Could you check a few things on this model? Use its own coordinates, in mm. Face numbers are marked on the shaded views. Round coordinates to 2 decimals unless told otherwise and drop trailing zeros. Loops run counter-clockwise (first coordinate to the right, second up) from the corner with the lowest first, then second, coordinate; pieces in that order, holes last. Notation, with made-up numbers: (10, 26) -> (18, 26) arc R29 cw to (18, 57) -> close; hole circle Ø9 at (-13, -28.5). An arc over 180 degrees is marked (long way). Put each result on its own line as item: value. Start each with the question number.
1. Imagine slicing it at A-A, the plane x = 3. Please give me the cut outline in (y, z) (3 decimals).
2. If we mould it in two halves opening along Z, with no side actions, what happens to the marked faces 1, 2 and 3? For each: pulls with the +Z half, pulls with the -Z half, needs draft (parallel to the pull), parting line crosses it, or undercut.
3. I need wall thicknesses on line 1 (Y direction, x = 1.9, z = 0) (3 decimals); line 2 (Y direction, x = 1.65, z = 1); line 3 (Z direction, x = 4.15, y = 0.25). Which ranges of each line are inside material? Lowest first, please. Write a range as [from, to].
4. I'm going to push flat-ended pins straight in: P1, Ø1, axis at x = 3.5, z = 0.5, coming from the +Y side; P2, Ø2, axis at x = 3.5, y = 1, coming from the +Z side; P3, Ø2, axis at x = 3.5, z = 2.5, coming from the -Y side; P4, Ø5, axis at y = 0, z = 0, coming from the +X side. Where does each tip first touch, or does it pass through?
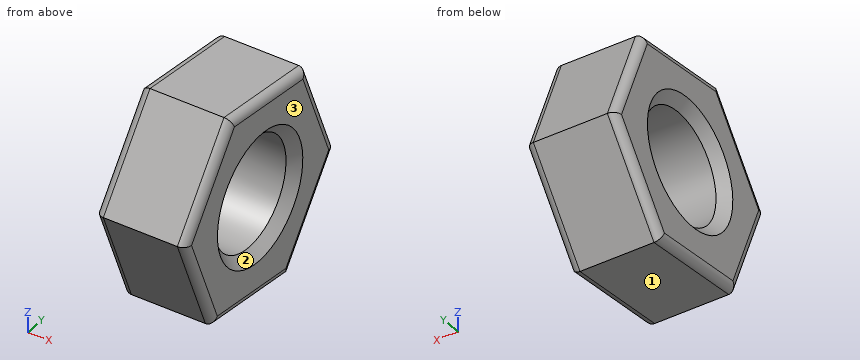
```python
from build123d import *

# Parameters (mm, degrees)
SKETCH1_R           = 2.705
BOSS_EXTRUDE1_DEPTH = 4.45
CHAMFER1_SIZE       = 0.5
FILLET1_R           = 0.4


with BuildPart() as part:
    # Sketch1 → Boss-Extrude1 (new body)
    with BuildSketch(Plane(origin=(0, 0, 0), x_dir=(0, 0, -1), z_dir=(1, 0, 0))):
        Polygon((0.806629144, 5.606072549), (-4.451686671, 3.501597604), (-5.258315815, -2.104474945), (-0.806629144, -5.606072549), (4.451686671, -3.501597604), (5.258315815, 2.104474945), align=None)
        Circle(SKETCH1_R, mode=Mode.SUBTRACT)
    extrude(amount=BOSS_EXTRUDE1_DEPTH)

    # Chamfer1
    chamfer1_edges = [part.edges().sort_by_distance(p)[0] for p in [
        (0, 0, 2.705),
        (4.45, 0, 2.705),
    ]]
    chamfer(chamfer1_edges, length=CHAMFER1_SIZE)

    # Fillet1
    fillet1_edges = [part.edges().sort_by_distance(p)[0] for p in [
        (4.45, 0.69856133, 4.855001243),
        (4.45, -3.855273747, 3.032472479),
        (4.45, -4.553835077, -1.822528764),
        (4.45, -0.69856133, -4.855001243),
        (4.45, 3.855273747, -3.032472479),
        (0, -0.69856133, -4.855001243),
        (0, -4.553835077, -1.822528764),
        (0, -3.855273747, 3.032472479),
        (0, 0.69856133, 4.855001243),
        (0, 4.553835077, 1.822528764),
        (0, 3.855273747, -3.032472479),
        (4.45, 4.553835077, 1.822528764),
    ]]
    fillet(fillet1_edges, radius=FILLET1_R)


solid = part.part
```
Entries:
1. outline: (-5.606, 0.807) -> (-3.502, -4.452) -> (2.104, -5.258) -> (5.606, -0.807) -> (3.502, 4.452) -> (-2.104, 5.258) -> close; hole circle Ø5.41 at (0, 0)
2. face 1: pulls with the -Z half
2. face 2: undercut
2. face 3: needs draft
3. line 1: [-5.283, -2.705], [2.705, 5.283]
3. line 2: [-5.45, -2.51], [2.51, 4.88]
3. line 3: [-4.98, -2.89], [2.89, 4.91]
4. P1: y = 5.28
4. P2: z = 4.96
4. P3: y = -5.06
4. P4: through
